Can you work these out from the model? Positions are in its coordinate system, mm. Face numbers are marked on the shaded views. A direction names the side the tool comes from. Give positions to 0.01 mm unless a question says otherwise; leave off trailing zeros. Loops run counter-clockwise (first coordinate to the right, second up) from the corner with the lowest first, then second, coordinate; pieces in that order, holes last. Notation, with made-up numbers: (6, 52) -> (33, 52) arc R13 ccw to (33, 59) -> close; hole circle Ø1 at (-23.75, 77). An arc over 180 degrees is marked (long way). One line per question, with ' | ' between items.
from build123d import *

# Parameters (mm, degrees)
SKETCH1_W           = 70
SKETCH1_H           = 50
BOSS_EXTRUDE1_DEPTH = 50
CUT_EXTRUDE1_DEPTH  = 50
CUT_EXTRUDE2_DEPTH  = 30
BOSS_EXTRUDE2_DEPTH = 30
SKETCH8_W           = 70
SKETCH8_H           = 40
CUT_EXTRUDE7_DEPTH  = 30
SKETCH9_W           = 70
SKETCH9_H           = 50
CUT_EXTRUDE8_DEPTH  = 30


with BuildPart() as part:
    # Sketch1 → Boss-Extrude1 (new body)
    with BuildSketch(Plane.XY):
        with Locations((35, 25)):
            Rectangle(SKETCH1_W, SKETCH1_H)
    extrude(amount=BOSS_EXTRUDE1_DEPTH)

    # Sketch2 → Cut-Extrude1 (cut)
    with BuildSketch(Plane.XY.offset(50)):
        Polygon((0, 40), (50, 40), (60, 50), (0, 50), align=None)
    extrude(amount=-CUT_EXTRUDE1_DEPTH, mode=Mode.SUBTRACT)

    # Sketch3 → Cut-Extrude2 (cut)
    with BuildSketch(Plane.XY.offset(50)):
        Polygon((50, 40), (30, 20), (30, 0), (0, 0), (0, 40), align=None)
    extrude(amount=-CUT_EXTRUDE2_DEPTH, mode=Mode.SUBTRACT)

    # Sketch7 → Boss-Extrude2 (add)
    with BuildSketch(Plane(origin=(0, 16, 32), x_dir=(-1, 0, 0), z_dir=(0, -0.447213595, -0.894427191))):
        Polygon((0, 26.83281573), (-50, 26.83281573), (-30, -17.88854382), (0, -17.88854382), align=None)
    extrude(amount=BOSS_EXTRUDE2_DEPTH)

    # Sketch8 → Cut-Extrude7 (cut)
    with BuildSketch(Plane(origin=(0, 0, 0), x_dir=(-1, 0, 0), z_dir=(0, 0, -1))):
        with Locations((-35, 20)):
            Rectangle(SKETCH8_W, SKETCH8_H)
    extrude(amount=CUT_EXTRUDE7_DEPTH, mode=Mode.SUBTRACT)

    # Sketch9 → Cut-Extrude8 (cut)
    with BuildSketch(Plane.XZ):
        with Locations((35, 25)):
            Rectangle(SKETCH9_W, SKETCH9_H)
    extrude(amount=CUT_EXTRUDE8_DEPTH, mode=Mode.SUBTRACT)


solid = part.part
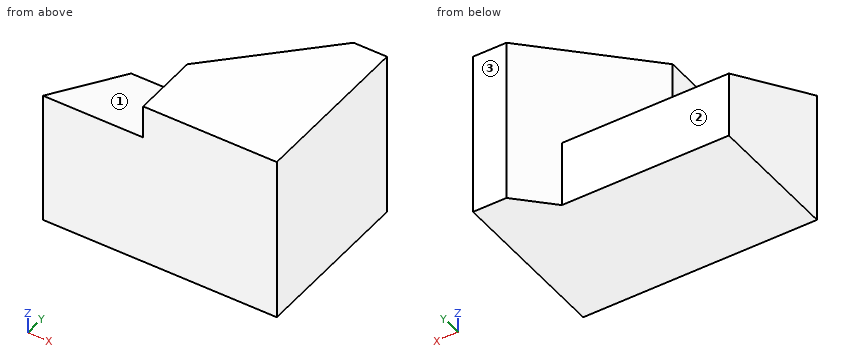
Q1. If we section it at B-B (y = 27.5): Write out the boundary of the cut face in (x, z).
Entries:
outline: (0, 0) -> (70, 0) -> (70, 50) -> (37.5, 50) -> (37.5, 26.25) -> (0, 26.25) -> close
Q2. If we section it at C-C (x = 38): Write out the boundary of the cut face in (y, z).
Entries:
outline: (0, 0) -> (40, 0) -> (40, 20) -> (28, 26) -> (28, 50) -> (0, 50) -> close
Q3. If I drill on probe 1 along Y at (x, z) = (42.5, 17.5); probe 2 along Y at (x, z) = (27, 29.5); probe 3 along X at (y, z) = (36, 26), over which ranges is the centre line in solid material (lowest first)? Write a range as from..to.
Entries:
probe 1: 0..40 | probe 2: 0..21 | probe 3: 46..70
Q4. On a 3-axis mill with a long thin cutter (end or side, diameter ignored), from which of +Z, -Z, +X, -X, +Y, -Y can I reach the whole of each face in a straight line? I mean the marked faces 1, 2 and 3. Say none if no direction works.
Entries:
face 1: +Z, -X, +Y | face 2: +Z, -Z, -X, +Y | face 3: +Z, -Z, +X, -X, +Y
Q5. For pin 1 Ø5 at (x, y) = (24, 6) entering from -Z; pin 2 Ø10 at (y, z) = (36, 31) entering from -X; pin 3 Ø6 at (x, z) = (27, 5.5) entering from +Y, each with a flat end and sliding along its axis, tell me the tip position at first contact or that it passes through.
Entries:
pin 1: z = 0 | pin 2: x = 41 | pin 3: y = 40
Q6. If we section it at D-D (y = 45.5): Write out the boundary of the cut face in (x, z).
Entries:
outline: (55.5, 0) -> (70, 0) -> (70, 50) -> (55.5, 50) -> close
Q7. If we section it at A-A (z = 38): Write out the boundary of the cut face in (x, y).
Entries:
outline: (0, 0) -> (70, 0) -> (70, 50) -> (60, 50) -> (30, 20) -> (30, 4) -> (0, 4) -> close
